The figure shows three views and two pictorial views of one solid part (mm, origin at its lowest corner). Answer the questions. A direction names the side the tool comes from. Give positions to 0.01 mm unless a question says otherwise; leave off trailing zeros. Loops run counter-clockwise (first coordinate to the right, second up) from the corner with the lowest first, then second, coordinate; pieces in that order, holes last. Notation, with made-up numbers: M -25,6 L 26,6 A35 ccw 26,43 Z; hole C -24,49.25 d10. An arc over 180 degrees is marked long. Answer in a Markdown table with one row per item. Add a question column.
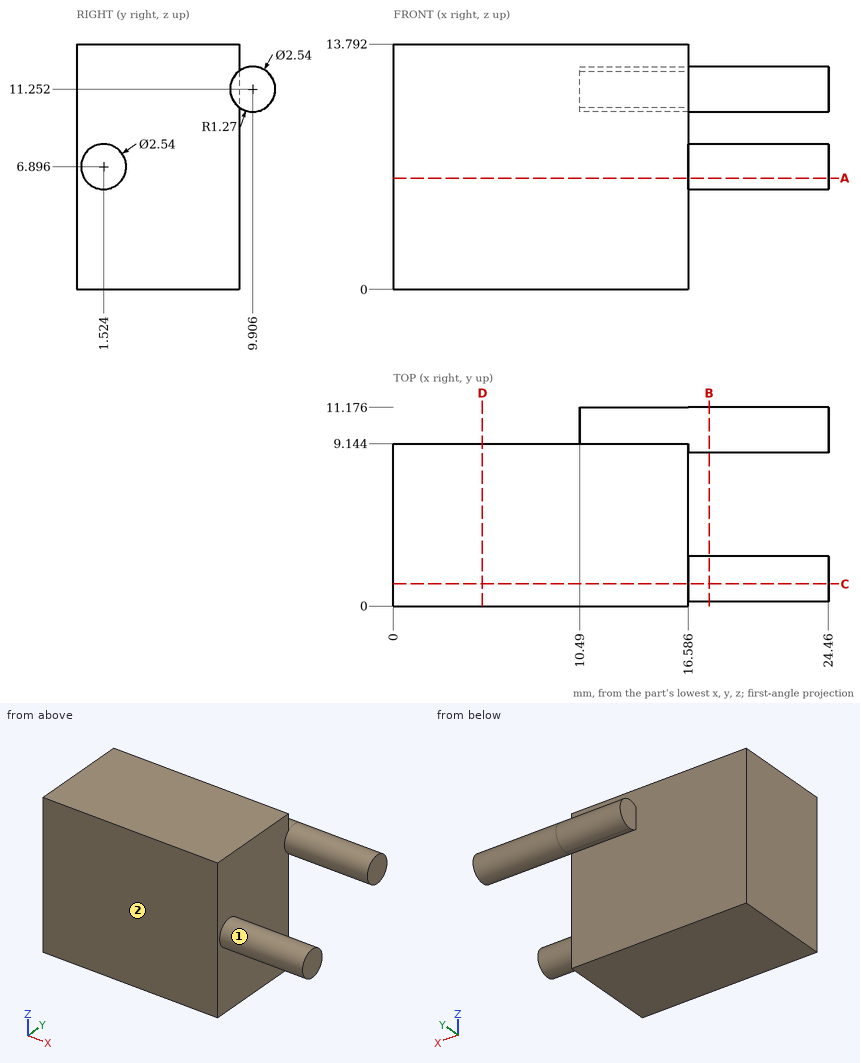
(1) Section A-A, the plane z = 6.25 is taken. Determine the outline of the cut face in (x, y).
(2) Which of the six approach directions +Z, -Z, +X, -X, +Y, -Y give full straight-line access (tool end or side, diameter ignored) to the marked faces 1 and 2?
(3) Consider line 1 along Y through (x, z) = (4.25, 11.5); line 2 along X through (y, z) = (3, 3.25); line 3 along Y through (x, z) = (14.5, 10.75). Determine where each line is inside the solid, lowest interval first. Write a range as from..to.
(4) Section B-B, the plane x = 17.75 is taken. Determine the outline of the cut face in (y, z).
(5) Each of these flat-tipped pins is pushed along its axis until it touches: P1, Ø2.5, axis at y = 6.5, z = 4.5, coming from the +X side; P2, Ø1.6, axis at y = 10, z = 11, coming from the -X side; P3, Ø8, axis at x = 9.5, z = 5.5, coming from the +Y side. Where does it stop, or does it pass through?
(6) Section C-C, the plane y = 1.25 is taken. Determine the outline of the cut face in (x, z), and give its area (3 significant figures).
(7) Section D-D, the plane x = 5 is taken. Determine the outline of the cut face in (y, z).
Numbers:
| question | item | result |
|---|---|---|
| 1 | outline | M 0,0 L 16.59,0 L 16.59,0.43 L 24.46,0.43 L 24.46,2.62 L 16.59,2.62 L 16.59,9.14 L 0,9.14 Z |
| 2 | face 1 | +X |
| 2 | face 2 | +Z, -Z, +X, -X, -Y |
| 3 | line 1 | y = 0..9.14 |
| 3 | line 2 | x = 0..16.59 |
| 3 | line 3 | y = 0..11.07 |
| 4 | outline | C 1.52,6.9 d2.54; C 9.91,11.25 d2.54 |
| 5 | P1 | stops at x = 16.59 |
| 5 | P2 | stops at x = 10.49 |
| 5 | P3 | stops at y = 9.14 |
| 6 | outline | M 0,0 L 16.59,0 L 16.59,5.66 L 24.46,5.66 L 24.46,8.14 L 16.59,8.14 L 16.59,13.79 L 0,13.79 Z |
| 6 | area | 248 mm² |
| 7 | outline | M 0,0 L 9.14,0 L 9.14,13.79 L 0,13.79 Z |
